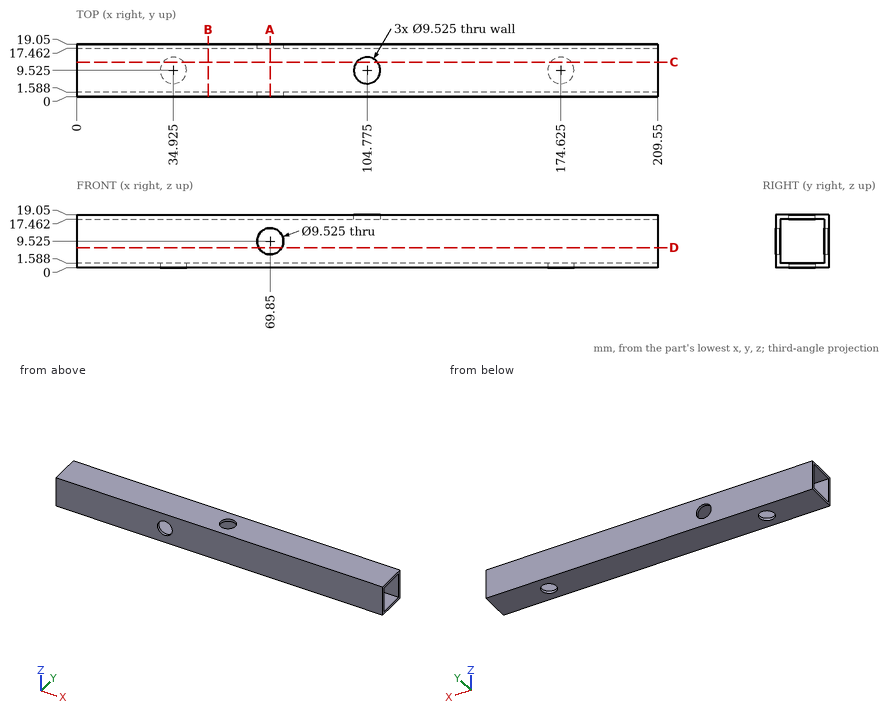
Part print with two shaded views. Sizes in mm from the minimum x, y, z corner. Round coordinates to 2 decimals unless told otherwise and drop trailing zeros. Order: outer loops, then holes, each group sorted by start corner. A loop starts at its lowest first (then second) coordinate and runs counter-clockwise, first axis right, second up. Notation, with made-up numbers: (-24.75, 52.5) -> (15.25, 52.5) arc R25 ccw to (15.25, 72.5) -> close; hole circle Ø1 at (-9.75, 11.5). An arc over 180 degrees is marked (long way). Write each question's results on one line, items separated by ' | '.
1. Cut at D-D (z = 7.25). Count the separate pieces of the cut face and the enclosed holes in it.
Findings below:
separate pieces: 4 | enclosed holes: 0
2. Cut at B-B (x = 47.5). Give the cut face in (y, z), plus the area to 3 significant figures.
Findings below:
outline: (0, 0) -> (19.05, 0) -> (19.05, 19.05) -> (0, 19.05) -> close; hole (1.59, 1.59) -> (17.46, 1.59) -> (17.46, 17.46) -> (1.59, 17.46) -> close | area: 111 mm²
3. Cut at A-A (x = 69.85). Give the cut face in (y, z).
Findings below:
outline: (0, 0) -> (19.05, 0) -> (19.05, 4.76) -> (17.46, 4.76) -> (17.46, 1.59) -> (1.59, 1.59) -> (1.59, 4.76) -> (0, 4.76) -> close; (0, 14.29) -> (1.59, 14.29) -> (1.59, 17.46) -> (17.46, 17.46) -> (17.46, 14.29) -> (19.05, 14.29) -> (19.05, 19.05) -> (0, 19.05) -> close
4. Flat gauge pin, fed straight in: P1, Ø5.5, axis at x = 174.625, y = 9.525, coming from the -Z side. Where does the tip first touch, or does it go through?
Findings below:
P1: stops at z = 17.46
5. Wall check: line 1 along Y through (x, z) = (170, 6.25); line 2 along Z through (x, y) = (69.85, 0.95). Give the ranges that are in metal, low to high. Write a range as [from, to].
Findings below:
line 1: y = [0, 1.59], [17.46, 19.05] | line 2: z = [0, 4.76], [14.29, 19.05]
6. Cut at C-C (y = 12.5). Give the cut face in (x, z).
Findings below:
outline: (0, 0) -> (31.21, 0) -> (31.21, 1.59) -> (0, 1.59) -> close; (0, 17.46) -> (101.06, 17.46) -> (101.06, 19.05) -> (0, 19.05) -> close; (38.64, 0) -> (170.91, 0) -> (170.91, 1.59) -> (38.64, 1.59) -> close; (108.49, 17.46) -> (209.55, 17.46) -> (209.55, 19.05) -> (108.49, 19.05) -> close; (178.34, 0) -> (209.55, 0) -> (209.55, 1.59) -> (178.34, 1.59) -> close
